from build123d import *

# Parameters (mm, degrees)
F0_W     = 28.842004016
F0_H     = 16.7503710836
F1_DEPTH = 42.672
F2_R     = 4.2924717139
F3_R     = 4.2926
F4_T     = -2.54


# Not quite as in the source:
# - a shell that OpenCascade refuses in one call is made with other operations: the cavity is built on its own and cut out


with BuildPart() as f1:
    # F0 (on Top) → F1 (new body)
    with BuildSketch(Plane.XY):
        Rectangle(F0_W, F0_H)
    extrude(amount=F1_DEPTH)

    # F2
    f2_edges = [f1.edges().sort_by_distance(p)[0] for p in [
        (-14.421002, -8.375186, 21.336),
        (14.421002, -8.375186, 21.336),
        (0, -8.375186, 0),
        (0, -8.375186, 42.672),
    ]]
    fillet(f2_edges, radius=F2_R)

    # F3
    f3_edges = [f1.edges().sort_by_distance(p)[0] for p in [
        (14.421002, 8.375186, 21.336),
        (-14.421002, 8.375186, 21.336),
        (0, 8.375186, 0),
        (0, 8.375186, 42.672),
    ]]
    fillet(f3_edges, radius=F3_R)

    # F4: a shell. OpenCascade refuses it in one call, so the cavity is built on its own and cut out:
    # the body offset inwards by the wall thickness, plus a prism from it out through each open face.
    f4_core = offset(f1.part, amount=F4_T, mode=Mode.PRIVATE)
    f4_exits = [f4_core.faces().sort_by_distance(p)[0] for p in [
        (0, -6.4e-05, 40.132),
    ]]
    add(f4_core, mode=Mode.SUBTRACT)
    extrude(f4_exits, amount=-F4_T, mode=Mode.SUBTRACT)


solid = f1.part
Design review of the part built by this model. Coordinates are the model's own, in mm. A direction names the side the tool comes from. Round coordinates to 2 decimals unless told otherwise and drop trailing zeros. Write each loop counter-clockwise with the first axis right and the second up, starting at its lowest first coordinate (ties: lowest second). Pieces come first, ordered by that corner, then holes. Notation, with made-up numbers: (-2.5, 2.5) - (54.5, 2.5) arc R9 cw to (54.5, 10.5) - close; hole circle Ø7 at (66, 58.5). An arc over 180 degrees is marked (long way). Use a Markdown table: item, result. Add a question column.
1. We need section D-D (y = -5). State the section outline as (x, z) points, then the cut area to 3 significant figures.
2. For faces 4 (the face through (-11.38, -5.31, 21.6)), 5 (the face through (-13.2, -7.08, 21.63)), 6 (the face through (-11.881, 0, 22)), list the 3-axis set-ups (+Z, -Z, +X, -X, +Y, -Y) from which the entire face can be reached by the end or side of a thin tool; tool diameter is ignored.
3. Mouldability with a two-part tool opening along Y and no side actions: class faces 1 (the face through (0.166, -5.335, 39.605)), 2 (the face through (0.2, -7.15, 1.29)), 3 (the face through (14.421, 0, 21)) as +Y half, -Y half, draft (parallel to the pull), parting line (faces both ways), or undercut.
4. Clearance check with flat-ended pins moving along their axes: pin 1 (6.5 mm diameter, centred on x = 3.5, y = 0, fed in from +Z); pin 2 (1 mm diameter, centred on y = -6.5, z = 19, fed in from +X); pin 3 (3 mm diameter, centred on x = -3, z = 41, fed in from -Y). State where each tip first meets the part, or that it passes through.
5. We need section B-B (y = -1.25). State the section outline as (x, z) points, then the cut area to 3 significant figures.
6. Wall thickness on probe 1 along Y at (x, z) = (0, 17); probe 2 along X at (y, z) = (-3.75, 35.5); probe 3 along Z at (x, y) = (11.75, -2.25): over which ranges is each line inside the solid? List them lowest first.
7. We need section C-C (x = -2.25). State the section outline as (y, z) points, then the cut area to 3 significant figures.
8. We need section A-A (z = 17.5). State the section outline as (x, y) points, then the cut area to 3 significant figures.
Output:
| question | item | result |
|---|---|---|
| 1 | outline | (-14.32, 0.1) - (14.32, 0.1) - (14.32, 42.57) - (-14.32, 42.57) - close; hole (-11.62, 2.8) - (11.62, 2.8) - (11.62, 39.87) - (-11.62, 39.87) - close |
| 1 | area | 355 mm2 |
| 2 | face 4 | none |
| 2 | face 5 | +Z, -Z, -X, -Y |
| 2 | face 6 | +Z |
| 3 | face 1 | undercut |
| 3 | face 2 | -Y half |
| 3 | face 3 | draft |
| 4 | pin 1 | stops at z = 2.54 |
| 4 | pin 2 | stops at x = 13.97 |
| 4 | pin 3 | stops at y = -8.23 |
| 5 | outline | (-14.42, 0) - (14.42, 0) - (14.42, 42.67) - (11.88, 42.67) - (11.88, 2.54) - (-11.88, 2.54) - (-11.88, 42.67) - (-14.42, 42.67) - close |
| 5 | area | 277 mm2 |
| 6 | probe 1 | y = -8.38 to -5.84, 5.84 to 8.38 |
| 6 | probe 2 | x = -14.42 to -11.88, 11.88 to 14.42 |
| 6 | probe 3 | z = 0 to 2.54 |
| 7 | outline | (-8.38, 4.29) arc R4.29 ccw to (-4.08, 0) - (4.08, 0) arc R4.29 ccw to (8.38, 4.29) - (8.38, 38.38) arc R4.29 ccw to (4.08, 42.67) - (4.08, 40.13) arc R1.75 cw to (5.84, 38.38) - (5.84, 4.29) arc R1.75 cw to (4.08, 2.54) - (-4.08, 2.54) arc R1.75 cw to (-5.84, 4.29) - (-5.84, 38.38) arc R1.75 cw to (-4.08, 40.13) - (-4.08, 42.67) arc R4.29 ccw to (-8.38, 38.38) - close |
| 7 | area | 242 mm2 |
| 8 | outline | (-14.42, -4.08) arc R4.29 ccw to (-10.13, -8.38) - (10.13, -8.38) arc R4.29 ccw to (14.42, -4.08) - (14.42, 4.08) arc R4.29 ccw to (10.13, 8.38) - (-10.13, 8.38) arc R4.29 ccw to (-14.42, 4.08) - close; hole (-11.88, -4.08) arc R1.75 ccw to (-10.13, -5.84) - (10.13, -5.84) arc R1.75 ccw to (11.88, -4.08) - (11.88, 4.08) arc R1.75 ccw to (10.13, 5.84) - (-10.13, 5.84) arc R1.75 ccw to (-11.88, 4.08) - close |
| 8 | area | 193 mm2 |
